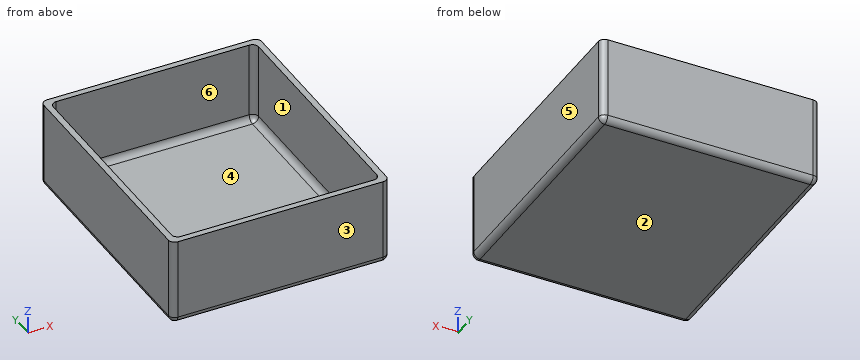
```python
from build123d import *

# Parameters (mm, degrees)
BOX003_W     = 66
BOX003_H     = 77
BOX003_DEPTH = 39
FILLET001_R  = 2
BOX002_W     = 70
BOX002_H     = 81
BOX002_DEPTH = 28
FILLET_R     = 2


with BuildPart() as bottomcut:
    # Box003 → Box003 (new body)
    with BuildSketch(Plane(origin=(2, 2, 2), x_dir=(1, 0, 0), z_dir=(0, 0, 1))):
        with Locations((33, 38.5)):
            Rectangle(BOX003_W, BOX003_H)
    extrude(amount=BOX003_DEPTH)

    # Fillet001
    fillet001_edges = [bottomcut.edges().sort_by_distance(p)[0] for p in [
        (2, 2, 21.5),
        (2, 79, 21.5),
        (2, 40.5, 2),
        (68, 2, 21.5),
        (68, 79, 21.5),
        (68, 40.5, 2),
        (35, 2, 2),
        (35, 79, 2),
    ]]
    fillet(fillet001_edges, radius=FILLET001_R)


with BuildPart() as bottom003:
    # Box002 → Box002 (new body)
    with BuildSketch(Plane.XY):
        with Locations((35, 40.5)):
            Rectangle(BOX002_W, BOX002_H)
    extrude(amount=BOX002_DEPTH)

    # Fillet
    fillet_edges = [bottom003.edges().sort_by_distance(p)[0] for p in [
        (0, 0, 14),
        (0, 81, 14),
        (0, 40.5, 0),
        (70, 0, 14),
        (70, 81, 14),
        (70, 40.5, 0),
        (35, 0, 0),
        (35, 81, 0),
    ]]
    fillet(fillet_edges, radius=FILLET_R)

    # Cut: cut bottomCut
    add(bottomcut.part, mode=Mode.SUBTRACT)


solid = bottom003.part
```
The model under review builds one solid part; all positions refer to its coordinate system, in mm. Face numbers are marked on the shaded views. A direction names the side the tool comes from. Round coordinates to 2 decimals unless told otherwise and drop trailing zeros. Order: outer loops, then holes, each group sorted by start corner. A loop starts at its lowest first (then second) coordinate and runs counter-clockwise, first axis right, second up. Notation, with made-up numbers: (67.25, 1.5) -> (117.25, 1.5) arc R7 cw to (117.25, 8.5) -> close; hole circle Ø10 at (-35, -32). An arc over 180 degrees is marked (long way). One line per item, written item: value. Start each with the question number.
Q1. Machinability: for the marked faces 1 and 2, which of the approach directions +Z, -Z, +X, -X, +Y, -Y give a long, thin tool a straight path to every point of the face, cutting with its end or side? Answer none if there is none.
Q2. Wall thickness on line 1 (Y direction, x = 27.5, z = 26.5); line 2 (X direction, y = 53, z = 19); line 3 (Z direction, x = 63, y = 16): over which ranges is each line inside the solid? List them lowest first.
Q3. Take a section at B-B (x = 47). Write out the cut boundary in (y, z).
Q4. Mouldability with a two-part tool opening along Y and no side actions: class the marked faces 3, 4, 5 and 6 as released by +Y, released by -Y, zero draft, split by the parting line, or undercut.
Q5. Take a section at A-A (z = 7.75). Write out the cut boundary in (x, y).
Q6. Take a section at C-C (y = 47.5). Write out the cut boundary in (x, z), and give its area (3 significant figures).
Reported:
1. face 1: +Z
1. face 2: -Z, +X, -X, +Y, -Y
2. line 1: y = 0 to 2, 79 to 81
2. line 2: x = 0 to 2, 68 to 70
2. line 3: z = 0 to 2
3. outline: (0, 2) arc R2 ccw to (2, 0) -> (79, 0) arc R2 ccw to (81, 2) -> (81, 28) -> (79, 28) -> (79, 4) arc R2 cw to (77, 2) -> (4, 2) arc R2 cw to (2, 4) -> (2, 28) -> (0, 28) -> close
4. face 3: released by -Y
4. face 4: undercut
4. face 5: zero draft
4. face 6: undercut
5. outline: (0, 2) arc R2 ccw to (2, 0) -> (68, 0) arc R2 ccw to (70, 2) -> (70, 79) arc R2 ccw to (68, 81) -> (2, 81) arc R2 ccw to (0, 79) -> close; hole (2, 4) arc R2 ccw to (4, 2) -> (66, 2) arc R2 ccw to (68, 4) -> (68, 77) arc R2 ccw to (66, 79) -> (4, 79) arc R2 ccw to (2, 77) -> close
6. outline: (0, 2) arc R2 ccw to (2, 0) -> (68, 0) arc R2 ccw to (70, 2) -> (70, 28) -> (68, 28) -> (68, 4) arc R2 cw to (66, 2) -> (4, 2) arc R2 cw to (2, 4) -> (2, 28) -> (0, 28) -> close
6. area: 244 mm2
